from build123d import *

# Parameters (mm, degrees)
BOSS_EXTRUDE1_DEPTH     = 15
CUT_EXTRUDE1_DEPTH      = 15
CUT_EXTRUDE1_DEPTH_BACK = 15


with BuildPart() as part:
    # Sketch1 → Boss-Extrude1 (new body)
    with BuildSketch(Plane(origin=(0, 0, 0), x_dir=(1, 0, 0), z_dir=(0, 1, 0))):
        with BuildLine():
            Line((-6.77549195, 3.313953488), (8.22450805, 3.313953488))
            Line((8.22450805, 3.313953488), (8.22450805, 1.813953488))
            Line((8.22450805, 1.813953488), (-3.27549195, 1.813953488))
            ThreePointArc((-3.27549195, 1.813953488), (-4.689705512, 1.228167051), (-5.27549195, -0.186046512))
            Line((-5.27549195, -0.186046512), (-5.27549195, -1.186046512))
            ThreePointArc((-5.27549195, -1.186046512), (-4.689705512, -2.600260074), (-3.27549195, -3.186046512))
            Line((-3.27549195, -3.186046512), (8.22450805, -3.186046512))
            Line((8.22450805, -3.186046512), (8.22450805, -4.686046512))
            Line((8.22450805, -4.686046512), (-6.77549195, -4.686046512))
            Line((-6.77549195, -4.686046512), (-6.77549195, -3.186046512))
            Line((-6.77549195, -3.186046512), (-6.77549195, 1.813953488))
            Line((-6.77549195, 1.813953488), (-6.77549195, 3.313953488))
        make_face()
    extrude(amount=BOSS_EXTRUDE1_DEPTH)

    # Sketch2 → Cut-Extrude1 (cut, two sides: drawn at the far end of the back side and taken through both)
    with BuildSketch(Plane(origin=(0, 0, 0), x_dir=(0, 0, -1), z_dir=(1, 0, 0)).offset(-CUT_EXTRUDE1_DEPTH_BACK)):
        Polygon((-3.186046512, 15), (3.313953488, 10), (3.313953488, 5), (-3.186046512, 0), (5.545494288, -1.974836629), (16.327123692, 9.034309621), (5.033464235, 17.721739972), align=None)
    extrude(amount=CUT_EXTRUDE1_DEPTH + CUT_EXTRUDE1_DEPTH_BACK, mode=Mode.SUBTRACT)


solid = part.part
The model under review builds one solid part; all positions refer to its coordinate system, in mm. A direction names the side the tool comes from. Give positions to 0.01 mm unless a question says otherwise; leave off trailing zeros. Loops run counter-clockwise (first coordinate to the right, second up) from the corner with the lowest first, then second, coordinate; pieces in that order, holes last. Notation, with made-up numbers: (81.5, 69) -> (96.5, 69) arc R15 ccw to (96.5, 75) -> close; hole circle Ø1 at (66, 20). An arc over 180 degrees is marked (long way). Write each question's results on one line, items separated by ' | '.
1) Take a section at A-A, the plane x = 0.25. Give the boundary of the cut face in (y, z), plus the area to 3 significant figures.
Conclusion:
outline: (0, 3.19) -> (15, 3.19) -> (15, 4.69) -> (0, 4.69) -> close; (3.85, -1.81) -> (5, -3.31) -> (10, -3.31) -> (11.15, -1.81) -> close | area: 31.7 mm^2
2) Take a section at D-D, the plane x = -4.5. Give the boundary of the cut face in (y, z).
Conclusion:
outline: (0, 3.19) -> (0.32, 2.77) -> (14.68, 2.77) -> (15, 3.19) -> (15, 4.69) -> (0, 4.69) -> close; (3.52, -1.4) -> (5, -3.31) -> (10, -3.31) -> (11.48, -1.4) -> close
3) Tool access review of faces 1 (the face through (1, 15, 4)), 2 (the face through (3, 7, -1.814)): name each direction out of +Z, -Z, +X, -X, +Y, -Y from which nothing blocks a thin tool from reaching the whole face with its end or side.
Conclusion:
face 1: +Z, -Z, +X, -X, +Y | face 2: +X, +Y, -Y
4) For line 1 along Z through (x, y) = (-2.5, 8.5); line 2 along Z through (x, y) = (3.5, 2); line 3 along X through (y, z) = (12.5, 1), list the stretches that pass through material, from the lowest coordinate up. Write a range as from..to.
Conclusion:
line 1: z = -3.31..-1.81, 3.19..4.69 | line 2: z = 3.19..4.69 | line 3: x = -6.78..-5.28
5) Draft analysis for pull direction Z (two halves, no side actions). For faces 3 (the face through (-5.275, 7, 1)), 4 (the face through (8.225, 7, -3)), 5 (the face through (-1.533, 3.993, -2.005)), 6 (the face through (1, 7, 4.686)), state which applies: pulls with the +Z half, pulls with the -Z half, needs draft (parallel to the pull), parting line crosses it, or undercut.
Conclusion:
face 3: undercut | face 4: needs draft | face 5: pulls with the -Z half | face 6: pulls with the +Z half
6) Take a section at B-B, the plane y = 6.5. Give the boundary of the cut face in (x, z), plus the area to 3 significant figures.
Conclusion:
outline: (-6.78, -3.31) -> (8.22, -3.31) -> (8.22, -1.81) -> (-3.28, -1.81) arc R2 cw to (-5.28, 0.19) -> (-5.28, 1.19) arc R2 cw to (-3.28, 3.19) -> (8.22, 3.19) -> (8.22, 4.69) -> (-6.78, 4.69) -> close | area: 54.2 mm^2
7) Take a section at C-C, the plane z = 3. Give the boundary of the cut face in (x, y).
Conclusion:
outline: (-6.78, 0.14) -> (-4.12, 0.14) -> (-4.12, 14.86) -> (-6.78, 14.86) -> close
8) Insertion check: pin 1 Ø4 at (x, z) = (2.5, -1.5) entering from -Y; pin 2 Ø0.8 at (y, z) = (9.5, 1) entering from +X; pin 3 Ø1 at (x, z) = (-1.5, 2) entering from +Y. Each pin has a flat end and moves straight along its axis. Give the tip position at first contact, or say it passes through.
Conclusion:
pin 1: stops at y = 3.85 | pin 2: stops at x = -5.26 | pin 3: passes through
